Geometry check sheet. Reference: the model listing, model coordinates, mm. Face numbers are marked on the shaded views. A direction names the side the tool comes from. Give positions to 0.01 mm unless a question says otherwise; leave off trailing zeros. Order: outer loops, then holes, each group sorted by start corner. A loop starts at its lowest first (then second) coordinate and runs counter-clockwise, first axis right, second up. Notation, with made-up numbers: M 33.5,-4.5 L 84.5,-4.5 A18 cw 84.5,7.5 Z; hole C 88.5,-32 d10. An arc over 180 degrees is marked long. One line per question, with ' | ' between items. Start each with the question number.
from build123d import *

# Parameters (mm, degrees)
SKETCH1_W           = 25
SKETCH1_H           = 10
SKETCH1_R           = 2.6
BOSS_EXTRUDE1_DEPTH = 5
SKETCH2_W           = 2
SKETCH2_H           = 15
BOSS_EXTRUDE2_DEPTH = 10


with BuildPart() as part:
    # Sketch1 → Boss-Extrude1 (new body)
    with BuildSketch(Plane(origin=(0, 0, 0), x_dir=(1, 0, 0), z_dir=(0, 1, 0))):
        Rectangle(SKETCH1_W, SKETCH1_H)
        with Locations(Location((-7.5, 0, 0), (0, 0, 270))):
            Circle(SKETCH1_R, mode=Mode.SUBTRACT)
        with Locations(Location((0, 0, 0), (0, 0, 270))):
            Circle(SKETCH1_R, mode=Mode.SUBTRACT)
        with Locations(Location((7.5, 0, 0), (0, 0, 270))):
            Circle(SKETCH1_R, mode=Mode.SUBTRACT)
    extrude(amount=BOSS_EXTRUDE1_DEPTH)

    # Sketch2 → Boss-Extrude2 (add)
    with BuildSketch(Plane.XY.offset(5)):
        with Locations((-13.5, -2.5)):
            Rectangle(SKETCH2_W, SKETCH2_H)
    extrude(amount=-BOSS_EXTRUDE2_DEPTH)


solid = part.part
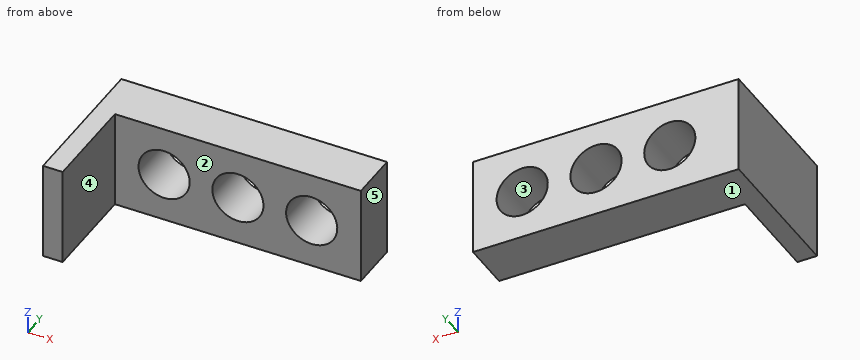
Item 1: Cross-section at C-C, the plane y = 0.5. Record the cut outline in (x, z), plus the area to 3 significant figures.
Item 2: Set-up check for the marked faces 4 and 5: record each of +Z, -Z, +X, -X, +Y, -Y from which the full face is reachable in a straight line by a thin tool's end or side.
Item 3: Mould release check, pull along Z, two halves, no side actions. Record for the marked faces 1, 2 and 3: released by +Z, released by -Z, zero draft, split by the parting line, or undercut.
Item 4: Cross-section at D-D, the plane x = -11. Record the cut outline in (y, z), plus the area to 3 significant figures.
Item 5: Cross-section at B-B, the plane z = 1. Record the cut outline in (x, y).
Item 6: Depth check by flat-ended pin: pin 1 (5 mm diameter, centred on y = -7, z = 2, fed in from +X); pin 2 (6 mm diameter, centred on x = 7.5, z = 0, fed in from +Y). Enter the tip coordinate at first touch or a pass-through.
Item 7: Cross-section at A-A, the plane x = -7.5. Record the cut outline in (y, z), plus the area to 3 significant figures.
Item 8: Material ranges on line 1 along X through (y, z) = (4, 0); line 2 along Y through (x, z) = (3, -4.5); line 3 along X through (y, z) = (-8.5, -3.25), recorded low to high.
Outcome:
1) outline: M -14.5,-5 L 12.5,-5 L 12.5,5 L -14.5,5 Z; hole C -7.5,0 d5.2; hole C 0,0 d5.2; hole C 7.5,0 d5.2 | area: 206 mm²
2) face 4: +Z, -Z, +X, -Y | face 5: +Z, -Z, +X, +Y, -Y
3) face 1: released by -Z | face 2: zero draft | face 3: undercut
4) outline: M 0,-5 L 5,-5 L 5,5 L 0,5 Z | area: 50.0 mm²
5) outline: M -14.5,-10 L -12.5,-10 L -12.5,0 L -9.9,0 L -9.9,5 L -14.5,5 Z; M -5.1,0 L -2.4,0 L -2.4,5 L -5.1,5 Z; M 2.4,0 L 5.1,0 L 5.1,5 L 2.4,5 Z; M 9.9,0 L 12.5,0 L 12.5,5 L 9.9,5 Z
6) pin 1: stops at x = -12.5 | pin 2: stops at y = 5
7) outline: M 0,-5 L 5,-5 L 5,-2.6 L 0,-2.6 Z; M 0,2.6 L 5,2.6 L 5,5 L 0,5 Z | area: 24.0 mm²
8) line 1: x = -14.5 to -10.1, -4.9 to -2.6, 2.6 to 4.9, 10.1 to 12.5 | line 2: y = 0 to 5 | line 3: x = -14.5 to -12.5
